Part model, mm, in its own coordinate system. Face numbers are marked on the shaded views. A direction names the side the tool comes from. Round coordinates to 2 decimals unless told otherwise and drop trailing zeros. Loops run counter-clockwise (first coordinate to the right, second up) from the corner with the lowest first, then second, coordinate; pieces in that order, holes last. Notation, with made-up numbers: M -32.75,-30.75 L 15.25,-30.75 A9 cw 15.25,-16.75 Z; hole C -31.75,-7.75 d3. An arc over 180 degrees is marked long. Put each result on its own line as item: value. Start each with the question number.
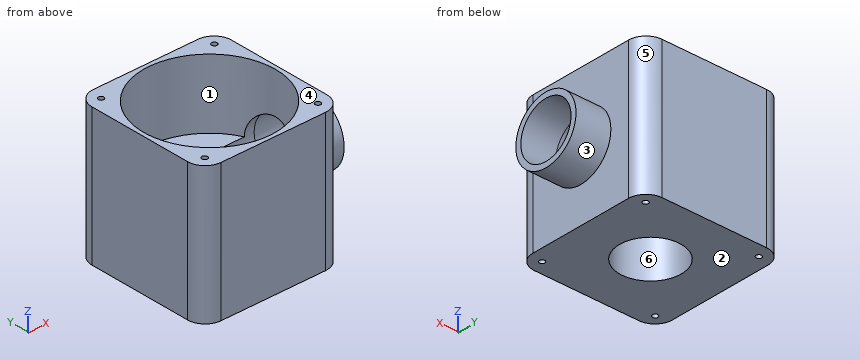
```python
from build123d import *

# Parameters (mm, degrees)
F0_W      = 101.6
F0_H      = 101.6
F0_R      = 48
F1_DEPTH  = 50
F2_R      = 20
F3_DEPTH  = 50.8
F4_R      = 48
F5_DEPTH  = 50
F6_R      = 22.5
F7_DEPTH  = 100.0010001
F8_R      = 24
F8_R_2    = 20
F9_DEPTH  = 25.4
F10_R     = 12.7
F12_D     = 4
F12_DEPTH = 15.6876
F12_TIP   = 1.2017212381
F14_D     = 4
F14_DEPTH = 15.7
F14_TIP   = 1.2017212381


with BuildPart() as f1:
    # F0 (on Top) → F1 (new body, symmetric)
    with BuildSketch(Plane.XY):
        Rectangle(F0_W, F0_H)
        Circle(F0_R, mode=Mode.SUBTRACT)
        Circle(F0_R)
    extrude(amount=F1_DEPTH, both=True)

    # F2 (on face) → F3 (cut)
    with BuildSketch(Plane.YZ.offset(50.8)):
        Circle(F2_R)
    extrude(amount=-F3_DEPTH, mode=Mode.SUBTRACT)

    # F4 (on face) → F5 (cut)
    with BuildSketch(Plane.XY.offset(50)):
        Circle(F4_R)
    extrude(amount=-F5_DEPTH, mode=Mode.SUBTRACT)

    # F6 (on face) → F7 (cut, through all)
    with BuildSketch(Plane(origin=(0, 0, -50), x_dir=(1, 0, 0), z_dir=(0, 0, -1))):
        Circle(F6_R)
    extrude(amount=-F7_DEPTH, mode=Mode.SUBTRACT)

    # F8 (on face) → F9 (join)
    with BuildSketch(Plane.YZ.offset(50.8)):
        Circle(F8_R)
        Circle(F8_R_2, mode=Mode.SUBTRACT)
    extrude(amount=F9_DEPTH)

    # F10
    f10_edges = [f1.edges().sort_by_distance(p)[0] for p in [
        (50.8, -50.8, 0),
        (-50.8, -50.8, 0),
        (50.8, 50.8, 0),
        (-50.8, 50.8, 0),
    ]]
    fillet(f10_edges, radius=F10_R)

    # F12
    with Locations(Plane.XY.offset(50)):
        with Locations((-41.275, 41.275), (41.275, 41.275), (41.275, -41.275), (-41.275, -41.275)):
            Hole(F12_D / 2, depth=F12_DEPTH)
            with Locations((0, 0, -(F12_DEPTH + F12_TIP / 2))):  # 118° drill point
                Cone(0, F12_D / 2, F12_TIP, mode=Mode.SUBTRACT)

    # F14
    with Locations(Plane(origin=(0, 0, -50), x_dir=(1, 0, 0), z_dir=(0, 0, -1))):
        with Locations((-41.275, 41.275), (41.275, 41.275), (-41.275, -41.275), (41.275, -41.275)):
            Hole(F14_D / 2, depth=F14_DEPTH)
            with Locations((0, 0, -(F14_DEPTH + F14_TIP / 2))):  # 118° drill point
                Cone(0, F14_D / 2, F14_TIP, mode=Mode.SUBTRACT)


solid = f1.part
```
1. Drop flat-ended pins along their axis: pin 1 (3 mm diameter, centred on x = -41.275, y = -41.275, fed in from -Z); pin 2 (2.5 mm diameter, centred on x = 41.275, y = 41.275, fed in from +Z); pin 3 (4 mm diameter, centred on x = 0.5, y = -24.5, fed in from +Z). Give the stop position or say it passes through.
2. Wall check: L1, parallel to Y at x = -1.5, z = 23.5; L2, parallel to X at y = 0, z = -34.5; L3, parallel to Z at x = 65, y = 1. Give the ranges that are in metal, low to high.
3. Cut at B-B, the plane y = 0. Give the cut face in (x, z), and give its area (3 significant figures).
4. Which spindle directions (+Z, -Z, +X, -X, +Y, -Y) get a long thin tool onto all of the face, cutting with end or side? Do the marked faces 1, 2 and 3. Say none if no direction does.
5. Cut at C-C, the plane z = -12. Give the cut face in (x, y).
6. Cut at D-D, the plane z = -41. Give the cut face in (x, y) (3 decimals), and give its area (3 significant figures).
7. Cut at A-A, the plane x = 0. Give the cut face in (y, z), and give its area (3 significant figures).
8. Mould opens along X. For the marked faces 4, 5 and 6 say: released by +X, released by -X, zero draft, split by the parting line, or undercut.
Results list:
1. pin 1: stops at z = -34
1. pin 2: stops at z = 33.86
1. pin 3: stops at z = 0
2. L1: y = -50.8 to -47.98, 47.98 to 50.8
2. L2: x = -50.8 to -22.5, 22.5 to 50.8
2. L3: z = -23.98 to -19.97, 19.97 to 23.98
3. outline: M -50.8,-50 L -22.5,-50 L -22.5,0 L -48,0 L -48,50 L -50.8,50 Z; M 22.5,-50 L 50.8,-50 L 50.8,-24 L 76.2,-24 L 76.2,-20 L 22.5,-20 Z; M 48,20 L 76.2,20 L 76.2,24 L 50.8,24 L 50.8,50 L 48,50 Z
3. area: 2,690 mm^2
4. face 1: +Z
4. face 2: -Z, +X, -X, +Y, -Y
4. face 3: +X
5. outline: M -50.8,-38.1 A12.7 ccw -38.1,-50.8 L 38.1,-50.8 A12.7 ccw 50.8,-38.1 L 50.8,-20.78 L 76.2,-20.78 L 76.2,-16 L 15.82,-16 A22.5 cw long 15.82,16 L 76.2,16 L 76.2,20.78 L 50.8,20.78 L 50.8,38.1 A12.7 ccw 38.1,50.8 L -38.1,50.8 A12.7 ccw -50.8,38.1 Z
6. outline: M -50.8,-38.1 A12.7 ccw -38.1,-50.8 L 38.1,-50.8 A12.7 ccw 50.8,-38.1 L 50.8,38.1 A12.7 ccw 38.1,50.8 L -38.1,50.8 A12.7 ccw -50.8,38.1 Z; hole C -41.275,-41.275 d4; hole C -41.275,41.275 d4; hole C 0,0 d45; hole C 41.275,-41.275 d4; hole C 41.275,41.275 d4
6. area: 8,540 mm^2
7. outline: M -50.8,-50 L -22.5,-50 L -22.5,0 L -48,0 L -48,50 L -50.8,50 Z; M 22.5,-50 L 50.8,-50 L 50.8,50 L 48,50 L 48,0 L 22.5,0 Z
7. area: 3,110 mm^2
8. face 4: zero draft
8. face 5: released by +X
8. face 6: undercut
